```python
from build123d import *

# Parameters (mm, degrees)
BOSS_EXTRUDE2_DEPTH      = 8
BOSS_EXTRUDE2_DEPTH_BACK = 8
SKETCH3_W                = 12.5
SKETCH3_H                = 5
SKETCH3_W_2              = 5.918941358
SKETCH3_H_2              = 2.496427957
CUT_EXTRUDE1_DEPTH       = 8
FILLET1_R                = 3
FILLET2_R                = 1
FILLET3_R                = 0.5


with BuildPart() as part:
    # Sketch2 → Boss-Extrude2 (new, two sides: drawn at the far end of the back side and taken through both)
    with BuildSketch(Plane(origin=(0, 0, 0), x_dir=(1, 0, 0), z_dir=(0, 1, 0)).offset(-BOSS_EXTRUDE2_DEPTH_BACK)):
        Polygon((-72.495595293, -0.799164043), (-72.495595293, 33.5), (72.495595293, 33.5), (71.070165431, -33.5), (-72.495595293, -33.5), align=None)
    extrude(amount=BOSS_EXTRUDE2_DEPTH + BOSS_EXTRUDE2_DEPTH_BACK)

    # Sketch3 → Cut-Extrude1 (cut)
    with BuildSketch(Plane.ZY.offset(72.495595293)):
        with Locations((-17.25, 0.071666465)):
            Rectangle(SKETCH3_W, SKETCH3_H)
        with Locations((17.25, 0.071666465)):
            Rectangle(SKETCH3_W, SKETCH3_H)
        with Locations((-0.029122914, 0.052810579)):
            Rectangle(SKETCH3_W_2, SKETCH3_H_2)
    extrude(amount=-CUT_EXTRUDE1_DEPTH, mode=Mode.SUBTRACT)

    # Fillet1
    fillet1_edges = [part.edges().sort_by_distance(p)[0] for p in [
        (71.782880362, -8, 0),
        (-72.495595293, 8, 0),
        (-0.712714931, 8, 33.5),
        (71.782880362, 8, 0),
        (0, 8, -33.5),
        (-0.712714931, -8, 33.5),
        (-72.495595293, -8, 0),
        (0, -8, -33.5),
        (-72.495595293, 0, 33.5),
        (71.070165431, 0, 33.5),
        (72.495595293, 0, -33.5),
        (-72.495595293, 0, -33.5),
    ]]
    fillet(fillet1_edges, radius=FILLET1_R)

    # Fillet2
    fillet2_edges = [part.edges().sort_by_distance(p)[0] for p in [
        (-72.495595293, -2.428333535, 17.25),
        (-72.495595293, 0.071666465, 23.5),
        (-72.495595293, 2.571666465, 17.25),
        (-72.495595293, 0.071666465, 11),
        (-72.495595293, 2.571666465, -17.25),
        (-72.495595293, 0.071666465, -23.5),
        (-72.495595293, -2.428333535, -17.25),
        (-72.495595293, 0.071666465, -11),
    ]]
    fillet(fillet2_edges, radius=FILLET2_R)

    # Fillet3
    fillet3_edges = [part.edges().sort_by_distance(p)[0] for p in [
        (-72.495595293, -1.1954034, -0.029122914),
        (-72.495595293, 0.052810578, 2.930347765),
        (-72.495595293, 1.301024557, -0.029122914),
        (-72.495595293, 0.052810578, -2.988593593),
    ]]
    fillet(fillet3_edges, radius=FILLET3_R)


solid = part.part
```
Design review of the part built by this model. Coordinates are the model's own, in mm. A direction names the side the tool comes from. Coordinates: 2 decimals unless noted, no trailing zeros.
1) For faces 4 (the cylindrical face through (-1.64, -7.14, 32.6)), 5 (the flat face through (-68, 0, -2.989)), 6 (the cylindrical face through (70.871, 7.145, 0.472)), list the 3-axis set-ups (+Z, -Z, +X, -X, +Y, -Y) from which the entire face can be reached by the end or side of a thin tool; tool diameter is ignored.
2) Clearance check with flat-ended pins moving along their axes: pin 1 (8 mm diameter, centred on y = 1, z = -13, fed in from +X); pin 2 (2.5 mm diameter, centred on y = -0.5, z = -16.5, fed in from -X); pin 3 (5.5 mm diameter, centred on y = -0.5, z = 15, fed in from -X). State where each tip first meets the part, or that it passes through.
3) Mouldability with a two-part tool opening along Z and no side actions: class faces 1 (the cylindrical face through (-71.64, 7.1, 0.43)), 2 (the flat face through (-68, 0, -23.5)), 3 (the cylindrical face through (0.94, 7.1, -32.64)) as +Z half, -Z half, draft (parallel to the pull), parting line (faces both ways), or undercut.
4) Wall thickness on line 1 along X through (y, z) = (-2, -6.5); line 2 along Y through (x, z) = (66, 31); line 3 along X through (y, z) = (-7, -10.5): over which ranges is each line inside the solid? List them lowest first.
Returned:
1. face 4: +Z, +X, -X, -Y
1. face 5: -X
1. face 6: +Z, +X, +Y
2. pin 1: stops at x = 72.14
2. pin 2: stops at x = -64.5
2. pin 3: stops at x = -72.48
3. face 1: draft
3. face 2: undercut
3. face 3: -Z half
4. line 1: x = -72.5 to 71.92
4. line 2: y = -7.96 to 7.96
4. line 3: x = -71.73 to 71.24
